from build123d import *

# Parameters (mm, degrees)
SKETCH_W             = 36
SKETCH_H             = 18
PAD_DEPTH            = 8
POCKET_DEPTH         = 18.001
POCKET001_DEPTH      = 18.001
POCKET001_DEPTH_BACK = 18.001
FILLET_R             = 2
THICKNESS_T          = -1
POCKET002_DEPTH      = 1


with BuildPart() as part:
    # Sketch → Pad (new body)
    with BuildSketch(Plane.XY):
        Rectangle(SKETCH_W, SKETCH_H)
    extrude(amount=PAD_DEPTH)

    # Sketch001 (on Face1 of Pad) → Pocket (cut, through all)
    with BuildSketch(Plane.XZ.offset(9)):
        Polygon((-18, 8), (-18, 0), (-16, 8), align=None)
        Polygon((18, 8), (18, 0), (16, 8), align=None)
    extrude(amount=-POCKET_DEPTH, mode=Mode.SUBTRACT)

    # Sketch002 → Pocket001 (cut, two sides)
    with BuildSketch(Plane.YZ) as pocket001_sk:
        Polygon((-9, 8), (-7, 8), (-9, 0), align=None)
        Polygon((9, 8), (7, 8), (9, 0), align=None)
    extrude(amount=-POCKET001_DEPTH, mode=Mode.SUBTRACT)
    extrude(pocket001_sk.sketch, amount=POCKET001_DEPTH_BACK, mode=Mode.SUBTRACT)

    # Fillet
    fillet_edges = [part.edges().sort_by_distance(p)[0] for p in [
        (-17, 8, 4),
        (-17, -8, 4),
        (17, -8, 4),
        (17, 8, 4),
    ]]
    fillet(fillet_edges, radius=FILLET_R)

    # Thickness
    thickness_openings = [part.faces().sort_by_distance(p)[0] for p in [
        (0, 0, 0),
    ]]
    offset(amount=THICKNESS_T, openings=thickness_openings, kind=Kind.INTERSECTION)

    # Sketch004 (on Face9 of Thickness) → Pocket002 (cut)
    with BuildSketch(Plane.XY.offset(8)):
        Polygon((-1.5, 3), (1.5, 3), (1.5, -3), (0.5, -3), (2.5, -5), (4.5, -3), (3.5, -3), (3.5, 5), (-1.5, 5), align=None)
    extrude(amount=-POCKET002_DEPTH, mode=Mode.SUBTRACT)


solid = part.part
Can you work these out from the model? Positions are in its coordinate system, mm. A direction names the side the tool comes from. Coordinates: 2 decimals unless noted, no trailing zeros. Write each loop counter-clockwise with the first axis right and the second up, starting at its lowest first coordinate (ties: lowest second). Pieces come first, ordered by that corner, then holes. Notation, with made-up numbers: (-6, 59.25) - (-2, 59.25) arc R12 ccw to (-2, 72.25) - close; hole circle Ø6 at (37, -12.75). An arc over 180 degrees is marked (long way). Return JSON: item names as keys, results as strings. Group by question number.
Item 1: We'd pull the mould along X, two halves only. Please class faces 4 (the face through (-16.424, -7.454, 3.997)), 5 (the face through (-1.5, 4, 7.5)), 6 (the face through (0, -8, 4)): pulls with the +X half, pulls with the -X half, needs draft (parallel to the pull), parting line crosses it, or undercut.
Item 2: If we section it at B-B (y = 4): Write out the boundary of the cut face in (x, z), then the cut area to 3 significant figures.
Item 3: Which directions (+Z, -Z, +X, -X, +Y, -Y) give clear straight access to the entire face, cutting with the end or side of a thin tool? Please do faces 1 (the face through (3.5, -4, 7.5)), 2 (the face through (-17, 0, 4)), 3 (the face through (-16.106, -0.098, 3.451)).
Item 4: Please list where these lines run through material, in increasing order: probe 1 along Z at (x, y) = (11, 1.75); probe 2 along X at (y, z) = (-3.25, 4.25); probe 3 along Y at (x, z) = (13, 1).
Item 5: If we section it at C-C (x = 12): Write out the boundary of the cut face in (y, z).
Item 6: I'm going to push flat-ended pins straight in: pin 1 Ø1.1 at (x, z) = (-0.5, 7.5) entering from +Y; pin 2 Ø0.8 at (y, z) = (0, 7.5) entering from -X (3 decimals); pin 3 Ø1.1 at (x, z) = (4, 7.5) entering from -Y; pin 4 Ø4 at (x, z) = (-2, 1.5) entering from -Y. Where does each tip first touch, or does it pass through?
Return value:
{
 "1": {"face 4": "pulls with the -X half", "face 5": "undercut", "face 6": "needs draft"},
 "2": {"outline": "(-18, 0) - (-16.97, 0) - (-15.22, 7) - (-1.5, 7) - (-1.5, 8) - (-16, 8) - close; (3.5, 7) - (15.22, 7) - (16.97, 0) - (18, 0) - (16, 8) - (3.5, 8) - close", "area": "41.7 mm^2"},
 "3": {"face 1": "+Z, -Z", "face 2": "+Z, -X, +Y, -Y", "face 3": "-Z"},
 "4": {"probe 1": "z = 7 to 8", "probe 2": "x = -16.94 to -15.91, 15.91 to 16.94", "probe 3": "y = -8.75 to -7.72, 7.72 to 8.75"},
 "5": {"outline": "(-9, 0) - (-7.97, 0) - (-6.22, 7) - (6.22, 7) - (7.97, 0) - (9, 0) - (7, 8) - (-7, 8) - close"},
 "6": {"pin 1": "stops at y = 7.26", "pin 2": "stops at x = -16.225", "pin 3": "stops at y = -7.26", "pin 4": "stops at y = -9"}
}
